Here's how the part is built. I have some questions about the finished solid (model axes, mm). A direction names the side the tool comes from. Give positions to 0.01 mm unless a question says otherwise; leave off trailing zeros. Write each loop counter-clockwise with the first axis right and the second up, starting at its lowest first coordinate (ties: lowest second). Pieces come first, ordered by that corner, then holes. Notation, with made-up numbers: (45, 12) -> (88, 12) arc R13 cw to (88, 25) -> close; hole circle Ø5 at (66, 37.5). An arc over 180 degrees is marked (long way). Return JSON: item names as keys, results as strings.
from build123d import *

# Parameters (mm, degrees)
BOSS_EXTRUDE1_DEPTH = 12
SKETCH3_W           = 20
SKETCH3_H           = 15
BOSS_EXTRUDE2_DEPTH = 1
SKETCH4_W           = 10
SKETCH4_H           = 10
BOSS_EXTRUDE3_DEPTH = 9
SKETCH5_R           = 2.5
BOSS_EXTRUDE7_DEPTH = 0.1


with BuildPart() as part:
    # Sketch1 → Boss-Extrude1 (new body)
    with BuildSketch(Plane(origin=(0, 0, 0), x_dir=(1, 0, 0), z_dir=(0, 1, 0))):
        Polygon((3, 2), (18, 2), (18, 13), (3, 13), (3, 11.8), (0, 11.8), (0, 15), (20, 15), (20, 0), (0, 0), (0, 6.7), (3, 6.7), align=None)
    extrude(amount=BOSS_EXTRUDE1_DEPTH)

    # Sketch3 → Boss-Extrude2 (add)
    with BuildSketch(Plane.XZ):
        with Locations((10, -7.5)):
            Rectangle(SKETCH3_W, SKETCH3_H)
    extrude(amount=BOSS_EXTRUDE2_DEPTH)

    # Sketch4 → Boss-Extrude3 (add)
    with BuildSketch(Plane.XZ.offset(1)):
        with Locations((15, -5)):
            Rectangle(SKETCH4_W, SKETCH4_H)
    extrude(amount=BOSS_EXTRUDE3_DEPTH)

    # Sketch5 → Boss-Extrude7 (add)
    with BuildSketch(Plane.ZY.offset(-18)):
        with Locations(Location((-10.49, 2.51, 0), (0, 0, 180))):
            Circle(SKETCH5_R)
    extrude(amount=BOSS_EXTRUDE7_DEPTH)


solid = part.part
1. Which directions (+Z, -Z, +X, -X, +Y, -Y) give clear straight access to the entire face, cutting with the end or side of a thin tool? Please do faces 4 (the face through (17.9, 2, -10)), 5 (the face through (10, -5, -5)), 6 (the face through (1, 6, -6.7)).
Taken from the geometry:
{"face 4": "+Y", "face 5": "+Z, -Z, -X, -Y", "face 6": "-X, +Y"}
2. Suppose I cut it at A-A, the plane x = 16.5. List the corners of the cut face in (y, z) for me.
Taken from the geometry:
{"outline": "(-10, -10) -> (-1, -10) -> (-1, -15) -> (12, -15) -> (12, -13) -> (0, -13) -> (0, -2) -> (12, -2) -> (12, 0) -> (-10, 0) -> close"}
3. Suppose I cut it at D-D, the plane x = 6.5. List the corners of the cut face in (y, z) for me, and give its area (3 significant figures).
Taken from the geometry:
{"outline": "(-1, -15) -> (12, -15) -> (12, -13) -> (0, -13) -> (0, -2) -> (12, -2) -> (12, 0) -> (-1, 0) -> close", "area": "63.0 mm²"}
4. For pin 1 Ø5 at (y, z) = (-7, -7) entering from -X; pin 2 Ø1.5 at (y, z) = (2.5, -11) entering from -X; pin 3 Ø6 at (x, z) = (5.5, -5) entering from -Y, each with a flat end and sliding along its axis, tell me the tip position at first contact or that it passes through.
Taken from the geometry:
{"pin 1": "stops at x = 10", "pin 2": "stops at x = 17.9", "pin 3": "stops at y = -1"}
5. If I drill on line 1 (Z direction, x = 14.5, y = 2.75); line 2 (Z direction, x = 2, y = 6.25); line 3 (X direction, y = 2, z = -2.5), over which ranges is the centre line in solid material (lowest first)? Write a range as [from, to].
Taken from the geometry:
{"line 1": "z = [-15, -13], [-2, 0]", "line 2": "z = [-15, -11.8], [-6.7, 0]", "line 3": "x = [0, 3], [18, 20]"}
6. If we mould it in two halves opening along X, with no side actions, what happens to faces 1 (the face through (0, 6, -6)), 2 (the face through (3, 6, -12)), 3 (the face through (10, 6, -15))? For each: released by +X, released by -X, zero draft, split by the parting line, or undercut.
Taken from the geometry:
{"face 1": "released by -X", "face 2": "undercut", "face 3": "zero draft"}
